Geometry check sheet. Reference: drawing and pictorial views, mm from the part's lowest x, y, z. A direction names the side the tool comes from. Give positions to 0.01 mm unless a question says otherwise; leave off trailing zeros. Loops run counter-clockwise (first coordinate to the right, second up) from the corner with the lowest first, then second, coordinate; pieces in that order, holes last. Notation, with made-up numbers: (11.5, 18.25) -> (49.5, 18.25) arc R24 ccw to (49.5, 33.25) -> close; hole circle Ø8 at (87.25, 18). An arc over 180 degrees is marked (long way). Write each question's results on one line, items separated by ' | '. Start each with the question number.
1. Gauge pin test, flat ends, axial feed: pin 1 Ø4 at (x, y) = (50, 13) entering from +Z; pin 2 Ø19 at (x, z) = (27.37, 27.37) entering from +Y; pin 3 Ø1.5 at (x, z) = (41.5, 51.5) entering from -Y; pin 4 Ø1.5 at (x, y) = (19, 13) entering from -Z. Record the tip position at first contact, or that the pin passes through.
2. Mould release check, pull along X, two halves, no side actions. Record for the marked faces 1, 2, 3 and 4: +X half, -X half, draft (parallel to the pull), parting line (faces both ways), or undercut.
3. Cross-section at B-B on x = 26.25. Record the boundary of the cut face in (y, z).
4. Cross-section at C-C on y = 8.75. Record the boundary of the cut face in (x, z).
5. Cross-section at A-A on z = 50. Count the separate pieces of the cut face and the enclosed holes in it.
6. Material ranges on L1, parallel to X at y = 10.9, z = 50; L2, parallel to Z at x = 73.75, y = 5.85 (1 decimal), recorded low to high. Write a range as from..to.
7. Tool access check on the marked faces 5 and 6. Record the directions out of +Z, -Z, +X, -X, +Y, -Y that give a thin tool (end or side, any length) a straight path to the whole face; none if there is none.
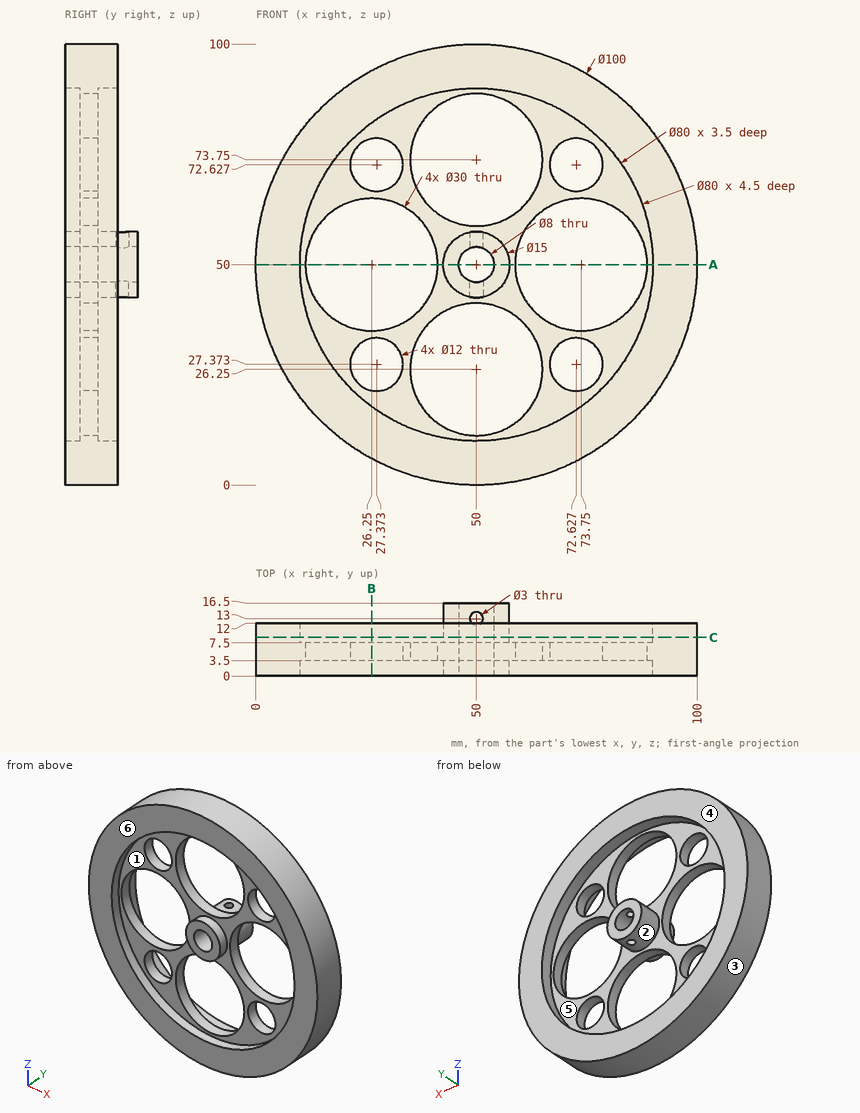
Geometry says:
1) pin 1: z = 100 | pin 2: y = 12 | pin 3: y = 3.5 | pin 4: through
2) face 1: undercut | face 2: undercut | face 3: parting line | face 4: draft
3) outline: (0, 6) -> (12, 6) -> (12, 17.81) -> (7.5, 17.81) -> (7.5, 21.48) -> (3.5, 21.48) -> (3.5, 17.81) -> (0, 17.81) -> close; (0, 82.19) -> (3.5, 82.19) -> (3.5, 78.52) -> (7.5, 78.52) -> (7.5, 82.19) -> (12, 82.19) -> (12, 94) -> (0, 94) -> close; (3.5, 33.27) -> (7.5, 33.27) -> (7.5, 35) -> (3.5, 35) -> close; (3.5, 65) -> (7.5, 65) -> (7.5, 66.73) -> (3.5, 66.73) -> close
4) outline: circle Ø100 at (50, 50); circle Ø15 at (50, 50); hole circle Ø80 at (50, 50); hole circle Ø8 at (50, 50)
5) separate pieces: 4 | enclosed holes: 0
6) L1: 0..10, 42.5..46, 54..57.5, 90..100 | L2: 6..21.5, 33.3..35, 65..66.7, 78.5..94
7) face 5: +Y | face 6: +Z, -Z, +X, -X, -Y
